from build123d import *

# Parameters (mm, degrees)
SKETCH_W        = 19.1
SKETCH_H        = 22
PAD_DEPTH       = 24
SKETCH001_W     = 22.8
SKETCH001_H     = 4.8
PAD001_DEPTH    = 24
SKETCH002_W     = 16.4
SKETCH002_H     = 18
POCKET_DEPTH    = 22
SKETCH003_W     = 8.2
SKETCH003_H     = 15
POCKET001_DEPTH = 5
SKETCH004_W     = 1.85
SKETCH004_H     = 2
SKETCH004_H_2   = 4.4
PAD002_DEPTH    = 20
SKETCH005_W     = 19.1
SKETCH005_H     = 4.4
PAD003_DEPTH    = 4


with BuildPart() as part:
    # Sketch → Pad (new body)
    with BuildSketch(Plane.XY):
        with Locations((-18.174118, 15.421817)):
            Rectangle(SKETCH_W, SKETCH_H)
    extrude(amount=PAD_DEPTH)

    # Sketch001 → Pad001 (new body)
    with BuildSketch(Plane.XY.offset(24)):
        with Locations((-18.174118, 19.121817)):
            Rectangle(SKETCH001_W, SKETCH001_H)
    extrude(amount=-PAD001_DEPTH)

    # Sketch002 → Pocket (cut)
    with BuildSketch(Plane.XY.offset(24)):
        with Locations((-18.174118, 13.421817)):
            Rectangle(SKETCH002_W, SKETCH002_H)
    extrude(amount=-POCKET_DEPTH, mode=Mode.SUBTRACT)

    # Sketch003 → Pocket001 (cut)
    with BuildSketch(Plane(origin=(0, 26.421817, 0), x_dir=(-1, 0, 0), z_dir=(0, 1, 0))):
        with Locations((19.824118, 10.5)):
            Rectangle(SKETCH003_W, SKETCH003_H)
    extrude(amount=-POCKET001_DEPTH, mode=Mode.SUBTRACT)

    # Sketch004 → Pad002 (new body)
    with BuildSketch(Plane.XY.offset(24)):
        with Locations((-25.449118, 5.421817)):
            Rectangle(SKETCH004_W, SKETCH004_H)
        with Locations((-10.899118, 5.421817)):
            Rectangle(SKETCH004_W, SKETCH004_H)
        with Locations((-25.449118, 13.321817)):
            Rectangle(SKETCH004_W, SKETCH004_H_2)
        with Locations((-10.899118, 13.321817)):
            Rectangle(SKETCH004_W, SKETCH004_H_2)
    extrude(amount=-PAD002_DEPTH)

    # Sketch005 → Pad003 (new body)
    with BuildSketch(Plane(origin=(0, 0, 0), x_dir=(1, 0, 0), z_dir=(0, 0, -1))):
        with Locations((-18.174118, -13.321817)):
            Rectangle(SKETCH005_W, SKETCH005_H)
    extrude(amount=-PAD003_DEPTH)


solid = part.part
The listing builds one solid part. Answer for the finished solid, in the listing's coordinates (mm). A direction names the side the tool comes from. Coordinates: 2 decimals unless noted, no trailing zeros. Order: outer loops, then holes, each group sorted by start corner. A loop starts at its lowest first (then second) coordinate and runs counter-clockwise, first axis right, second up. Notation, with made-up numbers: (80, 8.25) -> (99, 8.25) arc R28 ccw to (99, 38.25) -> close; hole circle Ø8 at (43.5, -15.5). An arc over 180 degrees is marked (long way). Answer in a Markdown table with one row per item. Add a question column.
Item 1: Determine the mould class of faces 1 (the face through (-11, 6.422, 14)), 2 (the face through (-8, 16.722, 12)), 3 (the face through (-24.524, 5, 14)), 4 (the face through (-27.724, 11, 12)) for opening direction X: +X half, -X half, draft (parallel to the pull), parting line (faces both ways), or undercut.
Item 2: Find section A-A (x = -20.75). Write down the section's boundary in (y, z), then the cut area to 3 significant figures.
Item 3: Find section C-C (y = 20.25). Write down the section's boundary in (x, z).
Item 4: Which of the six approach directions +Z, -Z, +X, -X, +Y, -Y give full straight-line access (tool end or side, diameter ignored) to faces 5 (the face through (-25, 11.122, 10)), 6 (the face through (-18, 13, 4)), 7 (the face through (-8.624, 24, 12)), 8 (the face through (-20, 24, 18))?
Item 5: Find section D-D (z = 21.25). Write down the section's boundary in (x, y), then the cut area to 3 significant figures.
Item 6: Each of these flat-tipped pins is pushed along its axis until it touches: P1, Ø0.6, axis at x = -25.5, y = 5, coming from the -Z side; P2, Ø2.5, axis at y = 23.5, z = 17.5, coming from the +X side; P3, Ø3.5, axis at x = -19, y = 17.5, coming from the +Z side; P4, Ø1.5, axis at y = 12, z = 21, coming from the -X side. Where does it stop, or does it pass through?
Item 7: Find the intervals of material crossed by L1, parallel to Y at x = -11.25, z = 19; L2, parallel to Z at x = -21.5, y = 23; L3, parallel to X at y = 10.5, z = 16, in increasing order. Write a range as from..to.
Result set:
| question | item | result |
|---|---|---|
| 1 | face 1 | undercut |
| 1 | face 2 | draft |
| 1 | face 3 | undercut |
| 1 | face 4 | -X half |
| 2 | outline | (4.42, 0) -> (26.42, 0) -> (26.42, 3) -> (22.42, 3) -> (22.42, 2) -> (15.52, 2) -> (15.52, 4) -> (11.12, 4) -> (11.12, 2) -> (4.42, 2) -> close; (22.42, 18) -> (26.42, 18) -> (26.42, 24) -> (22.42, 24) -> close |
| 2 | area | 80.8 mm² |
| 3 | outline | (-29.57, 0) -> (-6.77, 0) -> (-6.77, 24) -> (-9.97, 24) -> (-9.97, 2) -> (-26.37, 2) -> (-26.37, 24) -> (-29.57, 24) -> close |
| 4 | face 5 | +Z |
| 4 | face 6 | +Z, -Y |
| 4 | face 7 | +Z, -Z, +X, +Y |
| 4 | face 8 | +Y, -Y |
| 5 | outline | (-29.57, 16.72) -> (-27.72, 16.72) -> (-27.72, 4.42) -> (-24.52, 4.42) -> (-24.52, 6.42) -> (-26.37, 6.42) -> (-26.37, 11.12) -> (-24.52, 11.12) -> (-24.52, 15.52) -> (-26.37, 15.52) -> (-26.37, 22.42) -> (-9.97, 22.42) -> (-9.97, 15.52) -> (-11.82, 15.52) -> (-11.82, 11.12) -> (-9.97, 11.12) -> (-9.97, 6.42) -> (-11.82, 6.42) -> (-11.82, 4.42) -> (-8.62, 4.42) -> (-8.62, 16.72) -> (-6.77, 16.72) -> (-6.77, 21.52) -> (-8.62, 21.52) -> (-8.62, 26.42) -> (-27.72, 26.42) -> (-27.72, 21.52) -> (-29.57, 21.52) -> close |
| 5 | area | 166 mm² |
| 6 | P1 | stops at z = 0 |
| 6 | P2 | stops at x = -8.62 |
| 6 | P3 | stops at z = 2 |
| 6 | P4 | stops at x = -27.72 |
| 7 | L1 | y = 4.42..6.42, 11.12..15.52, 22.42..26.42 |
| 7 | L2 | z = 0..3, 18..24 |
| 7 | L3 | x = -27.72..-26.37, -9.97..-8.62 |
